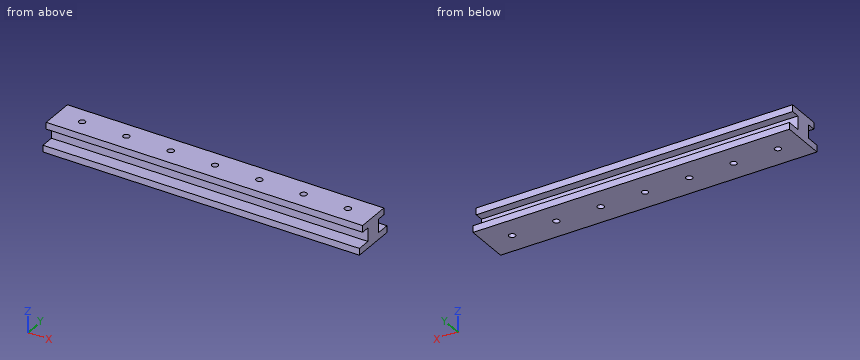
```python
from build123d import *

# Parameters (mm, degrees)
F0_W          = 150
F0_H          = 8
F1_DEPTH      = 6.35
F3_W          = 150
F3_H          = 16
F4_DEPTH      = 3.175
F5_W          = 150
F5_H          = 20.8
F6_DEPTH      = 3.175
F2_R          = 1.5
F7_DEPTH      = 25
F7_DEPTH_BACK = 20.1


with BuildPart() as f1:
    # F0 (on Top) → F1 (new body)
    with BuildSketch(Plane.XY):
        with Locations((75, 4)):
            Rectangle(F0_W, F0_H)
    extrude(amount=F1_DEPTH)

    # F3 (on face) → F4 (join)
    with BuildSketch(Plane.XY.offset(6.35)):
        with Locations((75, 4)):
            Rectangle(F3_W, F3_H)
    extrude(amount=F4_DEPTH)

    # F5 (on face) → F6 (join)
    with BuildSketch(Plane(origin=(0, 0, 0), x_dir=(1, 0, 0), z_dir=(0, 0, -1))):
        with Locations((75, -4)):
            Rectangle(F5_W, F5_H)
    extrude(amount=F6_DEPTH)

    # F2 (on face) → F7 (cut, two sides)
    with BuildSketch(Plane.XY.offset(6.35)) as f7_sk:
        with Locations((12, 4)):
            Circle(F2_R)
        with Locations((33, 4)):
            Circle(F2_R)
        with Locations((54, 4)):
            Circle(F2_R)
        with Locations((75, 4)):
            Circle(F2_R)
        with Locations((96, 4)):
            Circle(F2_R)
        with Locations((117, 4)):
            Circle(F2_R)
        with Locations((138, 4)):
            Circle(F2_R)
    extrude(amount=-F7_DEPTH, mode=Mode.SUBTRACT)
    extrude(f7_sk.sketch, amount=F7_DEPTH_BACK, mode=Mode.SUBTRACT)


solid = f1.part
```
Geometry: final body of the model. Coordinates: model frame, mm. Round coordinates to 2 decimals unless told otherwise and drop trailing zeros. Order: outer loops, then holes, each group sorted by start corner. A loop starts at its lowest first (then second) coordinate and runs counter-clockwise, first axis right, second up. Notation, with made-up numbers: (50, -39.75) -> (89, -39.75) arc R30 ccw to (89, -3.75) -> close; hole circle Ø9 at (26, -9.5). An arc over 180 degrees is marked (long way). Use one line per item in the form item = value. Start each with the question number.
1. Pin query (flat end, axial travel): pin 1 Ø1.8 at (x, y) = (12, 4) entering from -Z; pin 2 Ø3 at (x, z) = (32.5, 4.5) entering from +Y; pin 3 Ø1.6 at (x, z) = (42, 7.5) entering from +Y; pin 4 Ø1.9 at (x, z) = (67.5, 2) entering from -Y. Return the tip coordinate at first contact, or that it passes through.
2. Cut plane A-A (x = 96). Return the cut outline in (y, z) (3 decimals), then the cut area to 3 significant figures.
3. Cut plane C-C (z = 2.25). Return the cut outline in (x, y), then the cut area to 3 significant figures.
4. Cut plane B-B (y = 4). Count the separate pieces of the cut face and the enclosed holes in it, then the cut area to 3 significant figures.
5. Line query: probe 1 along Z at (x, y) = (116.5, 10.25) (3 decimals); probe 2 along Y at (x, z) = (33, 0.5); probe 3 along Y at (x, z) = (12, 6.75). Output: solid intervals per line, ascending.
Solution:
q1.pin_1 = through
q1.pin_2 = 8
q1.pin_3 = 12
q1.pin_4 = 0
q2.outline = (-6.4, -3.175) -> (2.5, -3.175) -> (2.5, 9.525) -> (-4, 9.525) -> (-4, 6.35) -> (0, 6.35) -> (0, 0) -> (-6.4, 0) -> close; (5.5, -3.175) -> (14.4, -3.175) -> (14.4, 0) -> (8, 0) -> (8, 6.35) -> (12, 6.35) -> (12, 9.525) -> (5.5, 9.525) -> close
q2.area = 130 mm^2
q3.outline = (0, 0) -> (150, 0) -> (150, 8) -> (0, 8) -> close; hole circle Ø3 at (12, 4); hole circle Ø3 at (33, 4); hole circle Ø3 at (54, 4); hole circle Ø3 at (75, 4); hole circle Ø3 at (96, 4); hole circle Ø3 at (117, 4); hole circle Ø3 at (138, 4)
q3.area = 1,150 mm^2
q4.separate_pieces = 8
q4.enclosed_holes = 0
q4.area = 1,640 mm^2
q5.probe_1 = -3.175 to 0, 6.35 to 9.525
q5.probe_2 = 0 to 2.5, 5.5 to 8
q5.probe_3 = -4 to 2.5, 5.5 to 12
